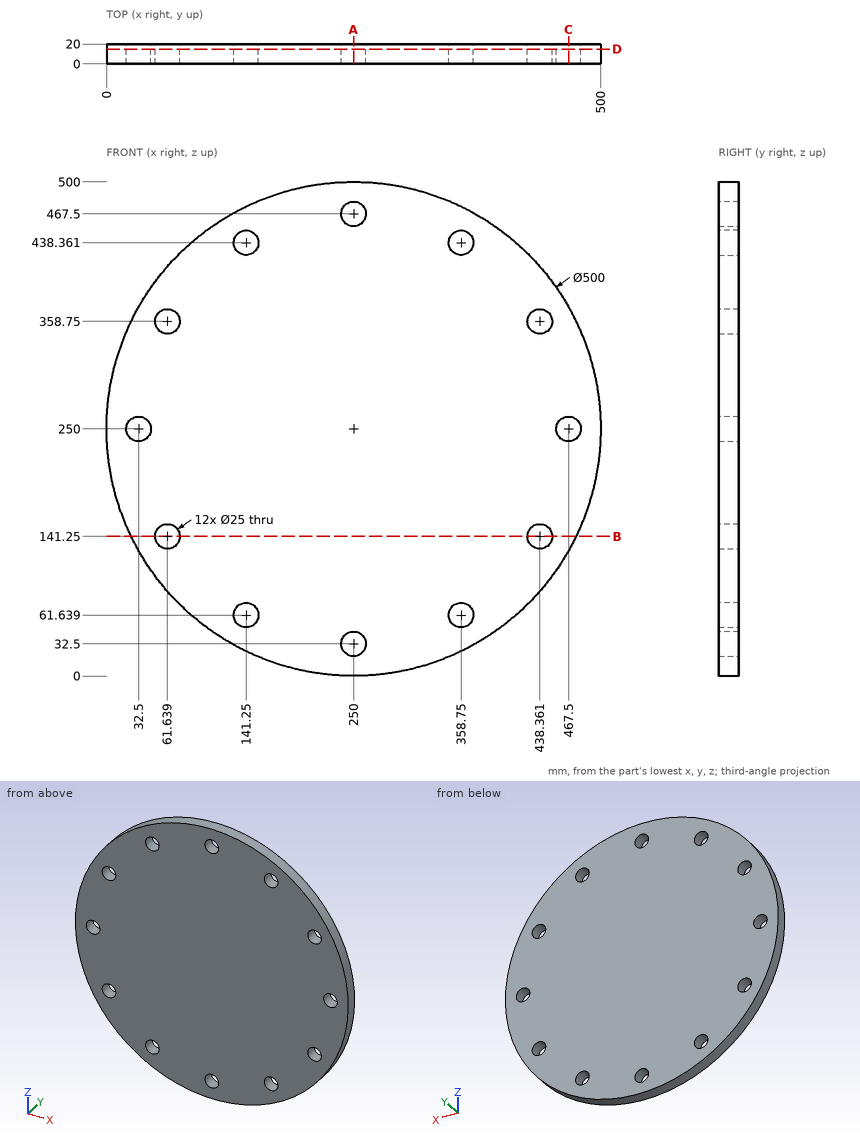
Geometry check sheet. Reference: drawing and pictorial views, mm from the part's lowest x, y, z. Give positions to 0.01 mm unless a question says otherwise; leave off trailing zeros. Write each loop counter-clockwise with the first axis right and the second up, starting at its lowest first coordinate (ties: lowest second). Pieces come first, ordered by that corner, then holes.
Item 1: Cross-section at C-C (x = 467.5). Enter the section's corners in (y, z), and give its area (3 significant figures).
Item 2: Cross-section at B-B (z = 141.25). Enter the section's corners in (x, y).
Item 3: Cross-section at D-D (y = 14.75). Count the separate pieces of the cut face and the enclosed holes in it, and give its area (3 significant figures).
Item 4: Gauge pin test, flat ends, axial feed: pin 1 (6 mm diameter, centred on x = 167.5, y = 2, fed in from -Z); pin 2 (1 mm diameter, centred on x = 103.5, y = 4, fed in from +Z); pin 3 (3 mm diameter, centred on x = 367, y = 7, fed in from -Z). Record the tip position at first contact, or that the pin passes through.
Item 5: Cross-section at A-A (x = 250). Enter the section's corners in (y, z).
Item 6: Scan lines: L1, parallel to X at y = 12.25, z = 250; L2, parallel to X at y = 15.25, z = 358.75; L3, parallel to Z at x = 69.5, y = 15.75 (1 decimal). Record each from-to range of solid material in increasing order.
Report:
1. outline: (0, 126.74) - (20, 126.74) - (20, 237.5) - (0, 237.5) - close; (0, 262.5) - (20, 262.5) - (20, 373.26) - (0, 373.26) - close
1. area: 4,430 mm2
2. outline: (24.89, 0) - (49.14, 0) - (49.14, 20) - (24.89, 20) - close; (74.14, 0) - (425.86, 0) - (425.86, 20) - (74.14, 20) - close; (450.86, 0) - (475.11, 0) - (475.11, 20) - (450.86, 20) - close
3. separate pieces: 1
3. enclosed holes: 12
3. area: 190,000 mm2
4. pin 1: stops at z = 12.98
4. pin 2: stops at z = 452.94
4. pin 3: stops at z = 28.28
5. outline: (0, 0) - (20, 0) - (20, 20) - (0, 20) - close; (0, 45) - (20, 45) - (20, 455) - (0, 455) - close; (0, 480) - (20, 480) - (20, 500) - (0, 500) - close
6. L1: x = 0 to 20, 45 to 455, 480 to 500
6. L2: x = 24.89 to 49.14, 74.14 to 425.86, 450.86 to 475.11
6. L3: z = 77 to 131.5, 151 to 349, 368.5 to 423
